Autodesk Inventor part; units mm, degrees
ref_plane "YZ Plane" through (0, 0, 0) normal (1, 0, 0) x (0, 1, 0)
ref_plane "XZ Plane" through (0, 0, 0) normal (0, 1, 0) x (-1, 0, 0)
ref_plane "XY Plane" through (0, 0, 0) normal (0, 0, 1) x (1, 0, 0)
sketch "Sketch2" plane through (0, 0, 0) normal (0, 1, 0) x (-1, 0, 0)
  line L0 (0, 0) -> (177.8, 0)
  line L1 (177.8, 0) -> (177.8, -203.2)
  line L2 (177.8, -203.2) -> (0, -203.2)
  line L3 (0, -203.2) -> (0, 0)
  dimension "d0" = 203.2
  dimension "d1" = 177.8
extrude "Extrusion1" add sketch "Sketch2" along normal blind 12.7
sketch "Sketch3" plane through (0, 12.7, 0) normal (0, 1, 0) x (1, 0, 0)
  line L0 (0, 0) -> (-177.8, 0)
  line L1 (-177.8, 0) -> (-177.8, 203.2)
  line L2 (-177.8, 203.2) -> (0, 203.2)
  line L3 (0, 203.2) -> (0, 0)
  line L4 (-171.45, 196.85) -> (-171.45, 6.35)
  line L5 (-171.45, 6.35) -> (-6.35, 6.35)
  line L6 (-6.35, 6.35) -> (-6.35, 196.85)
  line L7 (-6.35, 196.85) -> (-171.45, 196.85)
  dimension "d4" = 6.35
extrude "Extrusion2" add sketch "Sketch3" along normal blind 114.3
sketch "Sketch5" plane through (0, 12.7, 0) normal (0, 1, 0) x (1, 0, 0)
  line L0 (-63.5, 114.3) -> (-63.5, 6.35)
  line L1 (-6.35, 120.65) -> (-6.3512, 120.1928)
  line L2 (-171.45, 114.3) -> (-63.5, 114.3)
  line L3 (-171.45, 6.35) -> (-171.45, 196.85)
  line L4 (-6.35, 6.35) -> (-171.45, 6.35)
  line L5 (-171.45, 120.65) -> (-57.15, 120.65)
  line L6 (-57.15, 114.3) -> (-57.15, 6.35)
  line L7 (-171.45, 120.65) -> (-6.35, 120.65)
  line L8 (-57.15, 114.3) -> (-6.35, 114.3)
  line L9 (-6.35, 196.85) -> (-6.35, 6.35)
  line L10 (-171.45, 120.65) -> (-171.45, 114.3)
  line L11 (-6.35, 120.65) -> (-6.35, 114.3)
  line L12 (-6.35, 120.65) -> (-6.35, 114.3)
  line L13 (-63.5, 6.35) -> (-57.15, 6.35)
  line L14 (-171.45, 6.35) -> (-6.35, 6.35)
  dimension "d36" = 107.95
  dimension "d37" = 107.95
  dimension "d38" = 6.35
extrude "Extrusion5" add sketch "Sketch5" along normal blind 114.3 contours L2 L3 L5 L7 L1 L9 L8 L6 L4 L0
sketch "Sketch6" plane through (0, 0, 0) normal (0, -1, 0) x (1, 0, 0)
  line L0 (0, -203.2) -> (-177.8, 0) construction
  circle A0 centre (-88.9, -101.6) radius 101.6 construction
  line L1 (-177.8, -203.2) -> (0, 0) construction
  point P0 (-155.8041, -178.0618)
  point P1 (-155.8041, -25.1382)
  point P2 (-21.9959, -25.1382)
  point P3 (-21.9959, -178.0618)
  dimension "d25" = 203.2
hole "Hole1" at (-21.9959, 0, -25.1382) at (-155.8041, 0, -25.1382) at (-155.8041, 0, -178.0618) at (-21.9959, 0, -178.0618) direction (0, 1, 0) diameter 9.8044 end through all
sketch "Sketch7" plane through (-6.35, 12.7, -196.85) normal (-1, 0, 0) x (0, 0, 1)
  line L0 (76.2, 0) -> (0, 0)
  line L1 (76.2, 0) -> (76.2, 114.3)
  line L2 (0, 0) -> (76.2, 0)
  line L3 (76.2, 0) -> (76.2, 63.5)
  line L4 (76.2, 63.5) -> (0, 63.5)
  line L5 (0, 63.5) -> (0, 0)
  point P0 (196.85, -12.7)
  dimension "d39" = 63.5
extrude "Extrusion6" cut sketch "Sketch7" against normal blind 6.35
sketch "Sketch8" plane through (-177.8, 0, -203.2) normal (-1, 0, 0) x (0, 0, 1)
  line L0 (88.9, 12.7) -> (88.9, 127)
  line L1 (196.85, 127) -> (88.9, 127)
  line L2 (196.85, 12.7) -> (196.85, 127)
  line L3 (88.9, 12.7) -> (196.85, 12.7)
  point P0 (203.2, 0)
extrude "Extrusion7" cut sketch "Sketch8" against normal up to surface (114.3 mm away)
sketch "Sketch9" plane through (-177.8, 0, 0) normal (0, 0, 1) x (1, 0, 0)
  line L0 (0, 12.7) -> (114.3, 12.7)
  line L1 (114.3, 12.7) -> (114.3, 127)
  line L2 (0, 127) -> (114.3, 127)
  line L3 (0, 12.7) -> (0, 127)
  point P0 (177.8, 0)
extrude "Extrusion8" cut sketch "Sketch9" against normal up to surface (114.3 mm away)
sketch "Sketch10" plane through (0, 12.7, 0) normal (0, 1, 0) x (1, 0, 0)
  circle A0 centre (-155.8041, 25.1382) radius 4.9022
  line L0 (-177.8, 114.3) -> (-63.5, 114.3)
  line L1 (-177.8, 0) -> (-177.8, 114.3)
  line L2 (-63.5, 0) -> (-177.8, 0)
  line L3 (-63.5, 0) -> (-63.5, 114.3)
  line L4 (-177.8, 0) -> (-177.8, 114.3)
  line L5 (-6.35, 114.3) -> (-6.35, 6.35)
  line L6 (-6.35, 6.35) -> (-57.15, 6.35)
  line L7 (-57.15, 6.35) -> (-57.15, 114.3)
  line L8 (-57.15, 114.3) -> (-6.35, 114.3)
  line L9 (-171.45, 120.65) -> (-171.45, 196.85)
  line L10 (-171.45, 196.85) -> (-6.35, 196.85)
  line L11 (-6.35, 196.85) -> (-6.35, 120.65)
  line L12 (-6.35, 120.65) -> (-171.45, 120.65)
  line L13 (-63.5, 114.3) -> (-63.5, 0)
  line L14 (-63.5, 0) -> (0, 0)
  line L15 (0, 0) -> (0, 203.2)
  line L16 (0, 203.2) -> (-177.8, 203.2)
  line L17 (-177.8, 203.2) -> (-177.8, 114.3)
  line L18 (-177.8, 114.3) -> (-63.5, 114.3)
  point P0 (-177.8, 66.675)
extrude "Extrusion10" cut sketch "Sketch10" against normal through all contours L0 L3 L2 L1
properties part number "RSX Structure" material "Aluminum 6061"
For this review, take the finished solid that the model builds, in its own axes (mm). A direction names the side the tool comes from. Give positions to 0.01 mm unless a question says otherwise; leave off trailing zeros. Loops run counter-clockwise (first coordinate to the right, second up) from the corner with the lowest first, then second, coordinate; pieces in that order, holes last. Notation, with made-up numbers: M -23.5,39 L -16.5,39 A10 ccw -16.5,53 Z; hole C -39,-11.75 d7. An arc over 180 degrees is marked long. Put each result on its own line as item: value. Start each with the question number.
(1) Add section D-D, the plane y = 109. Write out the cut boundary in (x, z).
(2) For pin 1 (1 mm diameter, centred on y = 13.5, z = -44.5, fed in from -X); pin 2 (12 mm diameter, centred on x = -155, y = 40, fed in from +Z); pin 3 (15 mm diameter, centred on x = -38, z = -79, fed in from +Y), all flat-tipped, find the tip position at first contact; note any pin that passes through.
(3) The part is to be moulded in two halves that separate along X. For faces 1 (the flat face through (-68, 0, -123)), 2 (the flat face through (-57.15, 69, -61)), 3 (the flat face through (-177.8, 63, -158)), say which applies: +X half, -X half, draft (parallel to the pull), parting line (faces both ways), or undercut.
(4) Add section A-A, the plane z = -123.5. Write out the cut boundary in (x, y), then the cut area to 3 significant figures.
(5) Add section C-C, the plane y = 46.5. Write out the cut boundary in (x, z).
(6) Add section B-B, the plane x = -61. Write out the cut boundary in (y, z).
(7) Machinability: for faces 4 (the flat face through (-32, 69, -114.3)), 5 (the flat face through (-70, 127, -117)), 6 (the flat face through (-63.5, 64, -56)), 7 (the flat face through (-3, 76.2, -158)), which of the approach directions +Z, -Z, +X, -X, +Y, -Y give a long, thin tool a straight path to every point of the face, cutting with its end or side? Answer none if there is none.
(8) Wall thickness on L1, parallel to Z at x = -30, y = 48.5; L2, parallel to Z at x = -113, y = 26; L3, parallel to X at y = 107, z = -82.5: over which ranges is each line inside the solid? List them lowest first.
Result:
1. outline: M -177.8,-203.2 L 0,-203.2 L 0,0 L -63.5,0 L -63.5,-114.3 L -177.8,-114.3 Z; hole M -171.45,-196.85 L -6.35,-196.85 L -6.35,-120.65 L -171.45,-120.65 Z; hole M -57.15,-114.3 L -6.35,-114.3 L -6.35,-6.35 L -57.15,-6.35 Z
2. pin 1: stops at x = -63.5
2. pin 2: stops at z = -114.3
2. pin 3: stops at y = 12.7
3. face 1: draft
3. face 2: undercut
3. face 3: -X half
4. outline: M -177.8,0 L 0,0 L 0,12.7 L -171.45,12.7 L -171.45,127 L -177.8,127 Z; M -6.35,76.2 L 0,76.2 L 0,127 L -6.35,127 Z
4. area: 3,310 mm^2
5. outline: M -177.8,-203.2 L 0,-203.2 L 0,-196.85 L -171.45,-196.85 L -171.45,-120.65 L 0,-120.65 L 0,0 L -63.5,0 L -63.5,-114.3 L -177.8,-114.3 Z; hole M -57.15,-114.3 L -6.35,-114.3 L -6.35,-6.35 L -57.15,-6.35 Z
6. outline: M 0,-203.2 L 127,-203.2 L 127,-196.85 L 12.7,-196.85 L 12.7,-120.65 L 127,-120.65 L 127,0 L 0,0 Z
7. face 4: +Y
7. face 5: +Z, -Z, +X, -X, +Y
7. face 6: +Z, -X, +Y, -Y
7. face 7: +X
8. L1: z = -203.2 to -196.85, -120.65 to -114.3, -6.35 to 0
8. L2: z = -203.2 to -196.85, -120.65 to -114.3
8. L3: x = -63.5 to -57.15, -6.35 to 0
